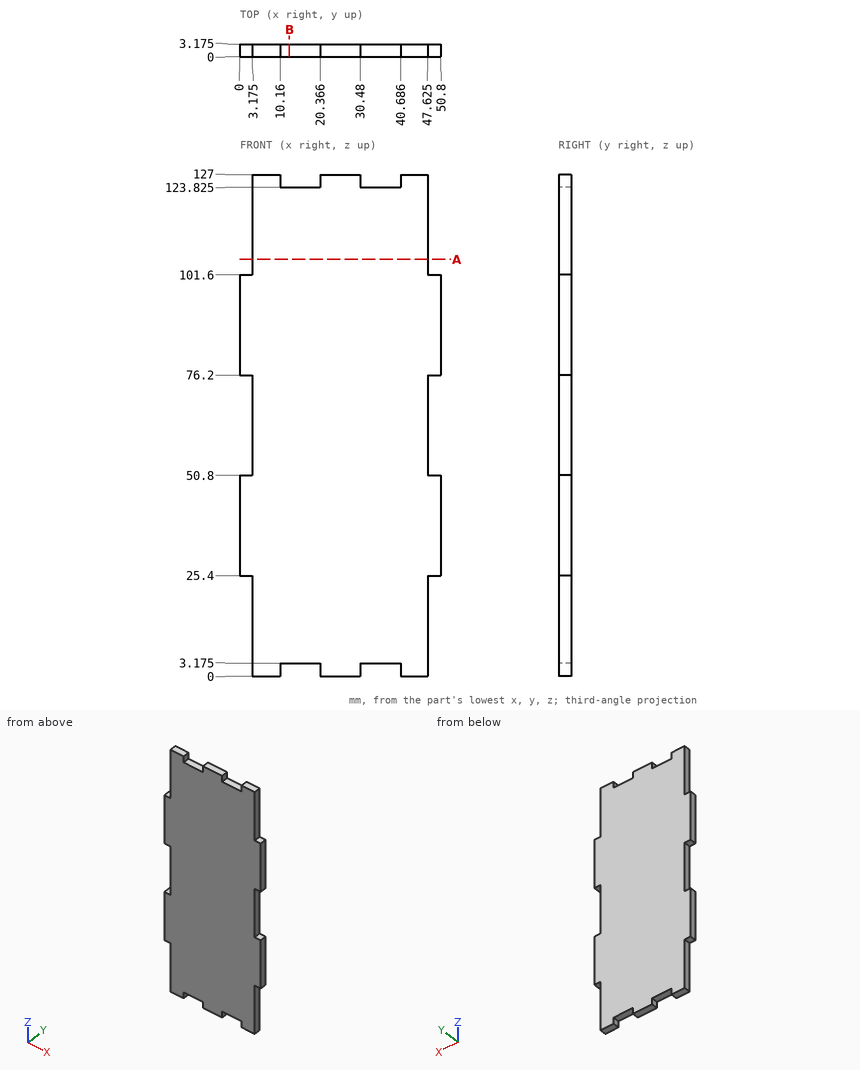
The drawing under review shows one solid part. Ordinate dimensions are in mm from its lowest x, y, z. Round coordinates to 2 decimals unless told otherwise and drop trailing zeros. Loops run counter-clockwise (first coordinate to the right, second up) from the corner with the lowest first, then second, coordinate; pieces in that order, holes last. Notation, with made-up numbers: (70.5, 30) - (97.5, 30) arc R11 cw to (97.5, 38) - close; hole circle Ø6 at (36.25, -35). An arc over 180 degrees is marked (long way). Put each result on its own line as item: value. Start each with the question number.
1. For probe 1 along Z at (x, y) = (3, 1.35); probe 2 along Z at (x, y) = (32.5, 2.25) (1 decimal); probe 3 along X at (y, z) = (2.2, 111) (1 decimal), list the stretches that pass through material, from the lowest coordinate up. Write a range as [from, to].
2. Insertion check: P1, Ø1.6, axis at y = 2, z = 125, coming from the +X side (3 decimals); P2, Ø1.6, axis at y = 2, z = 125.5, coming from the -X side (3 decimals); P3, Ø1, axis at x = 1.5, y = 1.5, coming from the -Z side. Each pin has a flat end and moves straight along its axis. Give the tip position at first contact, or say it passes through.
3. Consider section A-A on z = 105.5. State the section outline as (x, y) points (1 decimal), plus the area to 3 significant figures.
4. Consider section B-B on x = 12.5. State the section outline as (y, z) points (1 decimal), plus the area to 3 significant figures.
Result sheet:
1. probe 1: [25.4, 50.8], [76.2, 101.6]
1. probe 2: [3.2, 123.8]
1. probe 3: [3.2, 47.6]
2. P1: x = 47.625
2. P2: x = 3.175
2. P3: z = 25.4
3. outline: (3.2, 0) - (47.6, 0) - (47.6, 3.2) - (3.2, 3.2) - close
3. area: 141 mm^2
4. outline: (0, 3.2) - (3.2, 3.2) - (3.2, 123.8) - (0, 123.8) - close
4. area: 383 mm^2
